from build123d import *

# Parameters (mm, degrees)
SKIZZE1_W                       = 60
SKIZZE1_H                       = 60
AUFSATZ_LINEAR_AUSTRAGEN1_DEPTH = 5
SKIZZE7_R                       = 1.6
SCHNITT_LINEAR_AUSTRAGEN1_DEPTH = 10
FASE1_SIZE                      = 0.5
SKIZZE8_W                       = 25
SKIZZE8_H                       = 5
AUFSATZ_LINEAR_AUSTRAGEN2_DEPTH = 48
VERRUNDUNG3_R                   = 2.5


with BuildPart() as part:
    # Skizze1 → Aufsatz-Linear austragen1 (new body)
    with BuildSketch(Plane(origin=(0, 0, 0), x_dir=(1, 0, 0), z_dir=(0, 1, 0))):
        with Locations((25, 30)):
            Rectangle(SKIZZE1_W, SKIZZE1_H)
    extrude(amount=AUFSATZ_LINEAR_AUSTRAGEN1_DEPTH)

    # Skizze7 → Schnitt-Linear austragen1 (cut)
    with BuildSketch(Plane(origin=(0, 5, 0), x_dir=(1, 0, 0), z_dir=(0, 1, 0))):
        with Locations(Location((1.5, 53.5, 0), (0, 0, 270))):
            Circle(SKIZZE7_R)
        with Locations(Location((48.5, 53.5, 0), (0, 0, 270))):
            Circle(SKIZZE7_R)
        with Locations(Location((48.5, 6.5, 0), (0, 0, 270))):
            Circle(SKIZZE7_R)
        with Locations(Location((1.5, 6.5, 0), (0, 0, 270))):
            Circle(SKIZZE7_R)
    extrude(amount=-SCHNITT_LINEAR_AUSTRAGEN1_DEPTH, mode=Mode.SUBTRACT)

    # Fase1
    fase1_edges = [part.edges().sort_by_distance(p)[0] for p in [
        (-5, 2.5, -60),
        (55, 2.5, -60),
        (55, 2.5, 0),
        (-5, 2.5, 0),
    ]]
    chamfer(fase1_edges, length=FASE1_SIZE)

    # Skizze8 → Aufsatz-Linear austragen2 (add)
    with BuildSketch(Plane.XZ):
        with Locations((25, -30)):
            Rectangle(SKIZZE8_W, SKIZZE8_H)
    extrude(amount=AUFSATZ_LINEAR_AUSTRAGEN2_DEPTH)

    # Verrundung3
    verrundung3_edges = [part.edges().sort_by_distance(p)[0] for p in [
        (25, -48, -32.5),
        (25, -48, -27.5),
    ]]
    fillet(verrundung3_edges, radius=VERRUNDUNG3_R - 0.0001)  # a hair under: the kernel refuses the full size


solid = part.part
Read the model definition and answer for the solid it produces. Units are mm, in the model's axes. A direction names the side the tool comes from. Give positions to 0.01 mm unless a question says otherwise; leave off trailing zeros. Write each loop counter-clockwise with the first axis right and the second up, starting at its lowest first coordinate (ties: lowest second). Pieces come first, ordered by that corner, then holes. Notation, with made-up numbers: (80, -15) -> (126, -15) arc R11 cw to (126, -5) -> close; hole circle Ø7 at (89, 27.25). An arc over 180 degrees is marked (long way). Answer as a JSON object with one key per item and string values. Group by question number.
1) Find section A-A (z = -6.5). Write down the section's boundary in (x, y), and give its area (3 significant figures).
2) The mould has two halves that part along Z. Classify faces 6 (the flat face through (12.5, -24, -30)), 7 (the cylindrical face through (25, -47, -32)), 8 (the cylindrical face through (48.981, 2.535, -51.974)): +Z half, -Z half, draft (parallel to the pull), parting line (faces both ways), or undercut.
3) Consider L1, parallel to X at y = 3.1, z = -53.5; L2, parallel to X at y = 2, z = -53; L3, parallel to Z at x = 48, y = 4. Determine where each line is inside the solid, lowest interval first. Write a range as from..to.
4) Find section B-B (x = 48.5). Write down the section's boundary in (y, z).
5) Each of these flat-tipped pins is pushed along its axis until it touches: P1, Ø1, axis at x = 32, y = -9, coming from the -Z side; P2, Ø6, axis at x = 39, y = -22, coming from the +Z side; P3, Ø1.5, axis at y = -29.5, z = -30, coming from the +X side. Where does it stop, or does it pass through?
6) A tool of negligible diameter and unlimited length cuts with its end or side. For faces 1 (the cylindrical face through (49.85, 2.54, -5.64)), 2 (the flat face through (25, -22, -27.5)), 3 (the flat face through (25, 2, 0)), 4 (the flat face through (37.5, -24, -30)), 5 (the flat face through (25, -22, -32.5)), from which of +Z, -Z, +X, -X, +Y, -Y can it reach the whole face along a straight path? Write none if from no direction.
7) Find section D-D (y = -43). Write down the section's boundary in (x, z).
Values follow:
{
 "1": {"outline": "(-5, 0) -> (-0.1, 0) -> (-0.1, 5) -> (-5, 5) -> close; (3.1, 0) -> (46.9, 0) -> (46.9, 5) -> (3.1, 5) -> close; (50.1, 0) -> (55, 0) -> (55, 5) -> (50.1, 5) -> close", "area": "268 mm2"},
 "2": {"face 6": "draft", "face 7": "-Z half", "face 8": "undercut"},
 "3": {"L1": "x = -5..-0.1, 3.1..46.9, 50.1..55", "L2": "x = -5..-0.02, 3.02..46.98, 50.02..55", "L3": "z = -60..-55.02, -51.98..-8.02, -4.98..0"},
 "4": {"outline": "(0, -60) -> (5, -60) -> (5, -55.1) -> (0, -55.1) -> close; (0, -51.9) -> (5, -51.9) -> (5, -8.1) -> (0, -8.1) -> close; (0, -4.9) -> (5, -4.9) -> (5, 0) -> (0, 0) -> close"},
 "5": {"P1": "stops at z = -32.5", "P2": "stops at z = -27.5", "P3": "stops at x = 37.5"},
 "6": {"face 1": "+Y, -Y", "face 2": "+Z, +X, -X, -Y", "face 3": "+Z, +X, -X, +Y, -Y", "face 4": "+Z, -Z, +X, -Y", "face 5": "-Z, +X, -X, -Y"},
 "7": {"outline": "(12.5, -32.5) -> (37.5, -32.5) -> (37.5, -27.5) -> (12.5, -27.5) -> close"}
}
